Work out the finished part from the listing and answer in its coordinate system (mm). A direction names the side the tool comes from. Coordinates: 2 decimals unless noted, no trailing zeros. Loops run counter-clockwise (first coordinate to the right, second up) from the corner with the lowest first, then second, coordinate; pieces in that order, holes last. Notation, with made-up numbers: (54, -19.75) -> (113, -19.75) arc R7 ccw to (113, -12.75) -> close; hole circle Ø6 at (33.25, 8.5). An arc over 180 degrees is marked (long way). Answer as CSV lines item,"result".
```python
from build123d import *

# Parameters (mm, degrees)
SKETCH1_R           = 5.5
BOSS_EXTRUDE1_DEPTH = 4
BOSS_EXTRUDE4_DEPTH = 4
CHAMFER5_SIZE       = 2
CHAMFER5_SIZE2      = 0.69237056
CHAMFER6_SIZE       = 2
CHAMFER6_SIZE2      = 0.69237056
FILLET1_R           = 1
CIRPATTERN2_DEPTH   = 4


# Read off the part's stored shape, not the designer's step: CirPattern2
with BuildPart() as part:
    # Sketch1 → Boss-Extrude1 (new body)
    with BuildSketch(Plane(origin=(0, 0, 0), x_dir=(1, 0, 0), z_dir=(0, 1, 0))):
        with Locations(Location((0, 0, 0), (0, 0, 270))):
            Circle(SKETCH1_R)
        with BuildLine():
            Line((-1.51, -2.592276991), (-1.51, 2.592276991))
            ThreePointArc((-1.51, 2.592276991), (3, 0), (-1.51, -2.592276991))
        make_face(mode=Mode.SUBTRACT)
    extrude(amount=BOSS_EXTRUDE1_DEPTH)

    # Sketch2 → Boss-Extrude4 (add)
    with BuildSketch(Plane(origin=(0, 4, 0), x_dir=(1, 0, 0), z_dir=(0, 1, 0))):
        with BuildLine():
            Line((-4.906409736, 0.962882911), (-8, 1.57))
            Line((-8, 1.57), (-8, -1.57))
            Line((-8, -1.57), (-4.906409736, -0.962882911))
            ThreePointArc((-4.906409736, -0.962882911), (-5, 0), (-4.906409736, 0.962882911))
        make_face()
    extrude(amount=-BOSS_EXTRUDE4_DEPTH)

    # Chamfer5
    chamfer5_edges = [part.edges().sort_by_distance(p)[0] for p in [
        (-8, 2, -1.57),
    ]]
    chamfer5_side = [part.faces().sort_by_distance(p)[0] for p in [
        (-6.698525355, 2, -1.314585601),
    ]]
    chamfer(chamfer5_edges, length=CHAMFER5_SIZE, length2=CHAMFER5_SIZE2, reference=chamfer5_side[0])

    # Chamfer6
    chamfer6_edges = [part.edges().sort_by_distance(p)[0] for p in [
        (-8, 2, 1.57),
    ]]
    chamfer6_side = [part.faces().sort_by_distance(p)[0] for p in [
        (-6.698525355, 2, 1.314585601),
    ]]
    chamfer(chamfer6_edges, length=CHAMFER6_SIZE, length2=CHAMFER6_SIZE2, reference=chamfer6_side[0])

    # Fillet1
    fillet1_edges = [part.edges().sort_by_distance(p)[0] for p in [
        (-8, 2, -0.87762944),
        (-8, 2, 0.87762944),
    ]]
    fillet(fillet1_edges, radius=FILLET1_R)

    # CirPattern2 outline → CirPattern2 (add)
    with BuildSketch(Plane(origin=(0, 0, 0), x_dir=(1, 0, 0), z_dir=(0, 1, 0))):
        with BuildLine():
            ThreePointArc((-3.067344016, -4.565238295), (-3.889087297, -3.889087297), (-4.565238295, -3.067344016))
            Line((-4.565238295, -3.067344016), (-5.106925243, -3.431298779))
            Line((-5.106925243, -3.431298779), (-5.773253973, -4.344956726))
            ThreePointArc((-5.773253973, -4.344956726), (-5.962284465, -5.0117594), (-5.672403665, -5.641304834))
            Line((-5.672403665, -5.641304834), (-5.641304834, -5.672403665))
            ThreePointArc((-5.641304834, -5.672403665), (-5.0117594, -5.962284465), (-4.344956726, -5.773253973))
            Line((-4.344956726, -5.773253973), (-3.431298779, -5.106925243))
            Line((-3.431298779, -5.106925243), (-3.067344016, -4.565238295))
        make_face()
        with BuildLine():
            ThreePointArc((-4.565238295, 3.067344016), (-3.889087297, 3.889087297), (-3.067344016, 4.565238295))
            Line((-3.067344016, 4.565238295), (-3.431298779, 5.106925243))
            Line((-3.431298779, 5.106925243), (-4.344956726, 5.773253973))
            ThreePointArc((-4.344956726, 5.773253973), (-5.0117594, 5.962284465), (-5.641304834, 5.672403665))
            Line((-5.641304834, 5.672403665), (-5.672403665, 5.641304834))
            ThreePointArc((-5.672403665, 5.641304834), (-5.962284465, 5.0117594), (-5.773253973, 4.344956726))
            Line((-5.773253973, 4.344956726), (-5.106925243, 3.431298779))
            Line((-5.106925243, 3.431298779), (-4.565238295, 3.067344016))
        make_face()
        with BuildLine():
            ThreePointArc((-1.059171202, 5.39705071), (0, 5.5), (1.059171202, 5.39705071))
            Line((1.059171202, 5.39705071), (1.184846836, 6.037436105))
            Line((1.184846836, 6.037436105), (1.009958669, 7.154655399))
            ThreePointArc((1.009958669, 7.154655399), (0.672122719, 7.759820834), (0.021990194, 8))
            Line((0.021990194, 8), (-0.021990194, 8))
            ThreePointArc((-0.021990194, 8), (-0.672122719, 7.759820834), (-1.009958669, 7.154655399))
            Line((-1.009958669, 7.154655399), (-1.184846836, 6.037436105))
            Line((-1.184846836, 6.037436105), (-1.059171202, 5.39705071))
        make_face()
        with BuildLine():
            ThreePointArc((3.067344016, 4.565238295), (3.889087297, 3.889087297), (4.565238295, 3.067344016))
            Line((4.565238295, 3.067344016), (5.106925243, 3.431298779))
            Line((5.106925243, 3.431298779), (5.773253973, 4.344956726))
            ThreePointArc((5.773253973, 4.344956726), (5.962284465, 5.0117594), (5.672403665, 5.641304834))
            Line((5.672403665, 5.641304834), (5.641304834, 5.672403665))
            ThreePointArc((5.641304834, 5.672403665), (5.0117594, 5.962284465), (4.344956726, 5.773253973))
            Line((4.344956726, 5.773253973), (3.431298779, 5.106925243))
            Line((3.431298779, 5.106925243), (3.067344016, 4.565238295))
        make_face()
        with BuildLine():
            ThreePointArc((5.39705071, 1.059171202), (5.5, 0), (5.39705071, -1.059171202))
            Line((5.39705071, -1.059171202), (6.037436105, -1.184846836))
            Line((6.037436105, -1.184846836), (7.154655399, -1.009958669))
            ThreePointArc((7.154655399, -1.009958669), (7.759820834, -0.672122719), (8, -0.021990194))
            Line((8, -0.021990194), (8, 0.021990194))
            ThreePointArc((8, 0.021990194), (7.759820834, 0.672122719), (7.154655399, 1.009958669))
            Line((7.154655399, 1.009958669), (6.037436105, 1.184846836))
            Line((6.037436105, 1.184846836), (5.39705071, 1.059171202))
        make_face()
        with BuildLine():
            ThreePointArc((4.565238295, -3.067344016), (3.889087297, -3.889087297), (3.067344016, -4.565238295))
            Line((3.067344016, -4.565238295), (3.431298779, -5.106925243))
            Line((3.431298779, -5.106925243), (4.344956726, -5.773253973))
            ThreePointArc((4.344956726, -5.773253973), (5.0117594, -5.962284465), (5.641304834, -5.672403665))
            Line((5.641304834, -5.672403665), (5.672403665, -5.641304834))
            ThreePointArc((5.672403665, -5.641304834), (5.962284465, -5.0117594), (5.773253973, -4.344956726))
            Line((5.773253973, -4.344956726), (5.106925243, -3.431298779))
            Line((5.106925243, -3.431298779), (4.565238295, -3.067344016))
        make_face()
        with BuildLine():
            ThreePointArc((1.059171202, -5.39705071), (0, -5.5), (-1.059171202, -5.39705071))
            Line((-1.059171202, -5.39705071), (-1.184846836, -6.037436105))
            Line((-1.184846836, -6.037436105), (-1.009958669, -7.154655399))
            ThreePointArc((-1.009958669, -7.154655399), (-0.672122719, -7.759820834), (-0.021990194, -8))
            Line((-0.021990194, -8), (0.021990194, -8))
            ThreePointArc((0.021990194, -8), (0.672122719, -7.759820834), (1.009958669, -7.154655399))
            Line((1.009958669, -7.154655399), (1.184846836, -6.037436105))
            Line((1.184846836, -6.037436105), (1.059171202, -5.39705071))
        make_face()
    extrude(amount=CIRPATTERN2_DEPTH)


solid = part.part
```
(1) Flat-ended cylindrical pins translate along their axes: pin 1 Ø5 at (x, z) = (-4.5, 0.5) entering from -Y; pin 2 Ø1.5 at (x, y) = (4, 1) entering from +Z; pin 3 Ø2 at (x, z) = (1.5, -0.5) entering from +Y. Find the tip coordinate at first contact, or state that the pin passes through.
Computed values:
pin 1,"y = 0"
pin 2,"z = 5.95"
pin 3,"through"
(2) A cutting plane is placed at B-B, the plane x = 6.5. Write down the section's boundary in (y, z).
Computed values:
outline,"(0, -1.11) -> (4, -1.11) -> (4, 1.11) -> (0, 1.11) -> close"
(3) A cutting plane is placed at C-C, the plane z = 6.5. Write down the section's boundary in (x, y).
Computed values:
outline,"(-1.11, 0) -> (1.11, 0) -> (1.11, 4) -> (-1.11, 4) -> close"
(4) Which of the six approach directions +Z, -Z, +X, -X, +Y, -Y give full straight-line access (tool end or side, diameter ignored) to faces 1 (the face through (-3.89, 1.97, 5.44)), 2 (the face through (-5.435, 1.972, 3.882)), 3 (the face through (3.89, 1.97, -5.44))?
Computed values:
face 1,"+Z, +Y, -Y"
face 2,"-X, +Y, -Y"
face 3,"-Z, +Y, -Y"
(5) Consider line 1 along Z through (x, y) = (0, 1.5); line 2 along X through (y, z) = (0.35, 0.5); line 3 along X through (y, z) = (0.95, -2.5). Determine where each line is inside the solid, lowest interval first.
Computed values:
line 1,"-8 to -3, 3 to 8"
line 2,"-7.88 to -1.51, 2.96 to 7.88"
line 3,"-4.9 to -1.51, 1.66 to 4.9"
(6) For a pull along Z with two mould halves and no side action, classify faces 4 (the face through (-1.096, 1.972, -6.604)), 5 (the face through (-1.1, 1.97, 6.59)), 6 (the face through (-5.44, 1.97, -3.89)), 7 (the face through (-2, 4, 0)) as pulls with the +Z half, pulls with the -Z half, needs draft (parallel to the pull), parting line crosses it, or undercut.
Computed values:
face 4,"pulls with the -Z half"
face 5,"pulls with the +Z half"
face 6,"undercut"
face 7,"needs draft"
(7) A cutting plane is placed at A-A, the plane z = 0.25. Write down the section's boundary in (x, y), and give its area (3 significant figures).
Computed values:
outline,"(-7.97, 0) -> (-1.51, 0) -> (-1.51, 4) -> (-7.97, 4) -> close; (2.99, 0) -> (7.97, 0) -> (7.97, 4) -> (2.99, 4) -> close"
area,"45.8 mm2"
